For this review, use the dimensioned drawing (mm, ordinates from the lowest corner) and the shaded views. Give positions to 0.01 mm unless a question says otherwise; leave off trailing zeros. Order: outer loops, then holes, each group sorted by start corner. A loop starts at its lowest first (then second) coordinate and runs counter-clockwise, first axis right, second up. Notation, with made-up numbers: M 44.5,-12 L 101.5,-12 A12 ccw 101.5,2 Z; hole C -34.75,48 d2. An arc over 180 degrees is marked long. Answer as CSV lines item,"result". Start each with the question number.
1. We need section A-A, the plane z = 2.3. Give the boundary of the cut face in (x, y).
2. For line 1 along X through (y, z) = (10.5, 1.3) (1 decimal); line 2 along Y through (x, z) = (122, 1.6); line 3 along Y through (x, z) = (115, 0.35), list the stretches that pass through material, from the lowest coordinate up.
3. We need section C-C, the plane y = 2. Give the boundary of the cut face in (x, z), and give its area (3 significant figures).
4. We need section B-B, the plane x = 120. Give the boundary of the cut face in (y, z).
5. We need section D-D, the plane x = 74. Give the boundary of the cut face in (y, z).
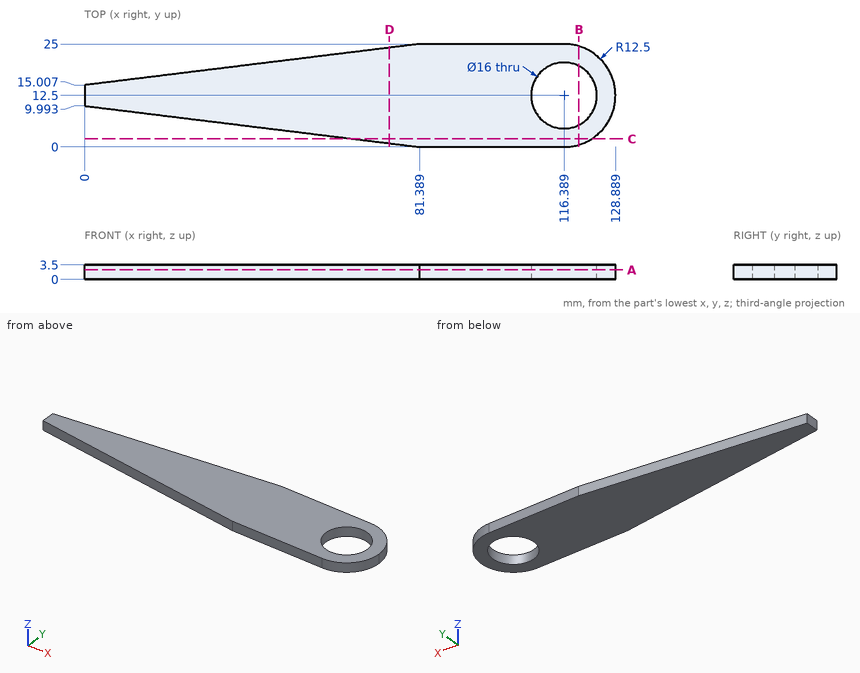
Result set:
1,outline,"M 0,9.99 L 81.39,0 L 116.39,0 A12.5 ccw 116.39,25 L 81.39,25 L 0,15.01 Z; hole C 116.39,12.5 d16"
2,line 1,"0 to 108.6, 124.1 to 128.7"
2,line 2,"1.33 to 6.8, 18.2 to 23.67"
2,line 3,"0 to 4.62, 20.38 to 25"
3,outline,"M 65.1,0 L 123.17,0 L 123.17,3.5 L 65.1,3.5 Z"
3,area,"203 mm2"
4,outline,"M 0.53,0 L 5.36,0 L 5.36,3.5 L 0.53,3.5 Z; M 19.64,0 L 24.47,0 L 24.47,3.5 L 19.64,3.5 Z"
5,outline,"M 0.91,0 L 24.09,0 L 24.09,3.5 L 0.91,3.5 Z"
